```python
from build123d import *

# Parameters (mm, degrees)
SKETCH1_R           = 1.5
BOSS_EXTRUDE1_DEPTH = 2


with BuildPart() as part:
    # Sketch1 → Boss-Extrude1 (new body)
    with BuildSketch(Plane(origin=(0, 0, 0), x_dir=(1, 0, 0), z_dir=(0, 1, 0))):
        with BuildLine():
            Line((-25, -16), (-12, -16))
            ThreePointArc((-12, -16), (0, -20), (12, -16))
            Line((12, -16), (25, -16))
            Line((25, -16), (25, 16))
            Line((25, 16), (12, 16))
            ThreePointArc((12, 16), (0, 20), (-12, 16))
            Line((-12, 16), (-25, 16))
            Line((-25, 16), (-25, -16))
        make_face()
        with BuildLine():
            Line((-22, 13), (-15.198684154, 13))
            ThreePointArc((-15.198684154, 13), (-20, 0), (-15.198684154, -13))
            Line((-15.198684154, -13), (-22, -13))
            Line((-22, -13), (-22, 13))
        make_face(mode=Mode.SUBTRACT)
        with BuildLine():
            ThreePointArc((15.198684154, -13), (20, 0), (15.198684154, 13))
            Line((15.198684154, 13), (22, 13))
            Line((22, 13), (22, -13))
            Line((22, -13), (15.198684154, -13))
        make_face(mode=Mode.SUBTRACT)
        with Locations(Location((0, 0, 0), (0, 0, 270))):
            Circle(SKETCH1_R, mode=Mode.SUBTRACT)
    extrude(amount=BOSS_EXTRUDE1_DEPTH)


solid = part.part
```
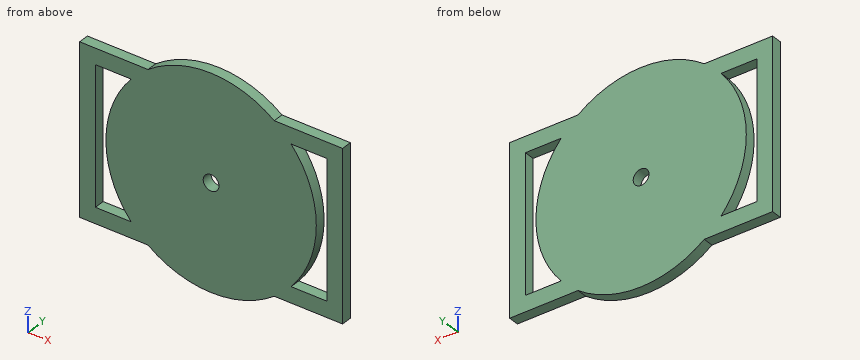
Model file for the job. Use its own axes, mm. Give positions to 0.01 mm unless a question says otherwise; leave off trailing zeros. Loops run counter-clockwise (first coordinate to the right, second up) from the corner with the lowest first, then second, coordinate; pieces in that order, holes last. Notation, with made-up numbers: M 37,9.25 L 65,9.25 A25 ccw 65,42.25 Z; hole C 78.5,30 d7. An arc over 180 degrees is marked long. Use one line per item in the form item = value.
Item 1: Drill centre lines: L1, parallel to X at y = 1.8, z = -12; L2, parallel to Z at x = 16.5, y = 0.8; L3, parallel to X at y = 0.2, z = 2. Where is each one in solid material? Low to high.
Filled in:
L1 = -25 to -22, -16 to 16, 22 to 25
L2 = -16 to -13, -11.3 to 11.3, 13 to 16
L3 = -25 to -22, -19.9 to 19.9, 22 to 25
Item 2: Slice it at C-C on y = 0.65. List the corners of the cut face in (x, z).
Filled in:
outline = M -25,-16 L -12,-16 A20 ccw 12,-16 L 25,-16 L 25,16 L 12,16 A20 ccw -12,16 L -25,16 Z; hole M -22,-13 L -15.2,-13 A20 cw -15.2,13 L -22,13 Z; hole C 0,0 d3; hole M 15.2,-13 L 22,-13 L 22,13 L 15.2,13 A20 cw Z
Item 3: Slice it at D-D on z = 6. List the corners of the cut face in (x, y), and give its area (3 significant figures).
Filled in:
outline = M -25,0 L -22,0 L -22,2 L -25,2 Z; M -19.08,0 L 19.08,0 L 19.08,2 L -19.08,2 Z; M 22,0 L 25,0 L 25,2 L 22,2 Z
area = 88.3 mm^2
Item 4: Flat gauge pins, fed straight in: pin 1 Ø10 at (x, z) = (-20, 7) entering from -Y; pin 2 Ø0.6 at (x, y) = (-17, 1) entering from +Z; pin 3 Ø1 at (x, y) = (18.5, 1) entering from -Z. Where does each tip first touch, or does it go through?
Filled in:
pin_1 = 0
pin_2 = 16
pin_3 = -16
Item 5: Slice it at B-B on z = 0. List the corners of the cut face in (x, y).
Filled in:
outline = M -25,0 L -22,0 L -22,2 L -25,2 Z; M -20,0 L -1.5,0 L -1.5,2 L -20,2 Z; M 1.5,0 L 20,0 L 20,2 L 1.5,2 Z; M 22,0 L 25,0 L 25,2 L 22,2 Z
Item 6: Slice it at A-A on x = 0. List the corners of the cut face in (y, z), and give its area (3 significant figures).
Filled in:
outline = M 0,-20 L 2,-20 L 2,-1.5 L 0,-1.5 Z; M 0,1.5 L 2,1.5 L 2,20 L 0,20 Z
area = 74.0 mm^2
